For this review, take the finished solid that the model builds, in its own axes (mm). Coordinates: 2 decimals unless noted, no trailing zeros.
1) Insertion check: P1, Ø3, axis at y = -3.5, z = 3.5, coming from the -X side. The pin has a flat end and moves straight along its axis. Give the tip position at first contact, or say it passes through.
2) To check wall thickness, follow line 1 along X through (y, z) = (17, 6.75); line 2 along Y through (x, z) = (-6, 0.5); line 3 along Y through (x, z) = (45, 2.5). State the ranges of each line that lie inside material, in increasing order.
3) Mouldability with a two-part tool opening along X and no side actions: class faces 1 (the face through (-9, 15, 8)), 2 (the face through (-8.796, -0.004, 3.944)) as pulls with the +X half, pulls with the -X half, needs draft (parallel to the pull), parting line crosses it, or undercut.
from build123d import *

# Parameters (mm, degrees)
BOSS_EXTRU_2_DEPTH                 = 8
ENL_V_MAT_EXTRU_1_DEPTH            = 9
CONG_1_R                           = 10
R_P_TITION_CIRCULAIRE1_COUNT       = 9
R_P_TITION_CIRCULAIRE1_ANGLE       = 3.68
CONG_1_OF_R_P_TITION_CIRCULAIRE1_R = 10
R_P_TITION_CIRCULAIRE2_COUNT       = 9
R_P_TITION_CIRCULAIRE2_ANGLE       = 3.68
CONG_1_OF_R_P_TITION_CIRCULAIRE2_R = 10


with BuildPart() as part:
    # Esquisse1 → Boss.-Extru.2 (new body)
    with BuildSketch(Plane.XY):
        with BuildLine():
            Line((627.808263697, -21.923547662), (631.296087384, 27.954654851))
            ThreePointArc((631.296087384, 27.954654851), (0, 50), (-631.296087384, 27.954654851))
            Line((-631.296087384, 27.954654851), (-627.808263697, -21.923547662))
            ThreePointArc((-627.808263697, -21.923547662), (0, 0), (627.808263697, -21.923547662))
        make_face()
    extrude(amount=BOSS_EXTRU_2_DEPTH)

    # Esquisse2 → Enlèv. mat.-Extru.1 (cut, through all)
    with BuildSketch(Plane.XY.offset(8)):
        Polygon((0, 25), (30, 49.950276106), (0, 74.995327729), (-30, 49.950276106), align=None)
    enl_v_mat_extru_1 = extrude(amount=-ENL_V_MAT_EXTRU_1_DEPTH, mode=Mode.SUBTRACT)

    # Congé1
    cong_1_edges = [part.edges().sort_by_distance(p)[0] for p in [
        (0, 25, 4),
        (-30, 49.950276106, 4),
        (30, 49.950276106, 4),
    ]]
    fillet(cong_1_edges, radius=CONG_1_R)

    # Répétition circulaire1: Enlèv. mat.-Extru.1 ×9 about axis
    r_p_tition_circulaire1_axis = Axis((0, -9000, 0), (0, 0, 1))
    for i in range(1, R_P_TITION_CIRCULAIRE1_COUNT):
        add(enl_v_mat_extru_1.rotate(r_p_tition_circulaire1_axis, i * R_P_TITION_CIRCULAIRE1_ANGLE / (R_P_TITION_CIRCULAIRE1_COUNT - 1)), mode=Mode.SUBTRACT)

    # Congé1 of Répétition circulaire1
    cong_1_of_r_p_tition_circulaire1_edges = [part.edges().sort_by_distance(p)[0] for p in [
        (-72.456565501, 24.709139142, 4),
        (-102.655910154, 49.417758293, 4),
        (-42.657843855, 49.899463992, 4),
        (-144.908460692, 23.836575317, 4),
        (-175.305203447, 48.301944876, 4),
        (-115.312938126, 49.265325224, 4),
        (-217.351015561, 22.382364766, 4),
        (-247.943197144, 46.602907776, 4),
        (-187.960599706, 48.047900678, 4),
        (-289.779560701, 20.346601223, 4),
        (-320.565209242, 44.320756509, 4),
        (-260.596145965, 46.247268824, 4),
        (-362.189427606, 17.729415908, 4),
        (-393.166558764, 41.455638174, 4),
        (-333.214895057, 43.863545726, 4),
        (-434.575948977, 14.530977515, 4),
        (-465.742566067, 38.007737447, 4),
        (-405.812166217, 40.89688503, 4),
        (-506.934459016, 10.751492204, 4),
        (-538.288553142, 33.977276569, 4),
        (-478.383280064, 37.347477958, 4),
        (-579.260293733, 6.39120359, 4),
        (-610.799843913, 29.364515329, 4),
        (-550.923558903, 33.215553293, 4),
    ]]
    fillet(cong_1_of_r_p_tition_circulaire1_edges, radius=CONG_1_OF_R_P_TITION_CIRCULAIRE1_R)

    # Répétition circulaire2: Enlèv. mat.-Extru.1 ×9 about axis
    r_p_tition_circulaire2_axis = Axis((0, -9000, 0), (0, 0, -1))
    for i in range(1, R_P_TITION_CIRCULAIRE2_COUNT):
        add(enl_v_mat_extru_1.rotate(r_p_tition_circulaire2_axis, i * R_P_TITION_CIRCULAIRE2_ANGLE / (R_P_TITION_CIRCULAIRE2_COUNT - 1)), mode=Mode.SUBTRACT)

    # Congé1 of Répétition circulaire2
    cong_1_of_r_p_tition_circulaire2_edges = [part.edges().sort_by_distance(p)[0] for p in [
        (72.456565501, 24.709139142, 4),
        (42.657843855, 49.899463992, 4),
        (102.655910154, 49.417758293, 4),
        (144.908460692, 23.836575317, 4),
        (115.312938126, 49.265325224, 4),
        (175.305203447, 48.301944876, 4),
        (217.351015561, 22.382364766, 4),
        (187.960599706, 48.047900678, 4),
        (247.943197144, 46.602907776, 4),
        (289.779560701, 20.346601223, 4),
        (260.596145965, 46.247268824, 4),
        (320.565209242, 44.320756509, 4),
        (362.189427606, 17.729415908, 4),
        (333.214895057, 43.863545726, 4),
        (393.166558764, 41.455638174, 4),
        (434.575948977, 14.530977515, 4),
        (405.812166217, 40.89688503, 4),
        (465.742566067, 38.007737447, 4),
        (506.934459016, 10.751492204, 4),
        (478.383280064, 37.347477958, 4),
        (538.288553142, 33.977276569, 4),
        (579.260293733, 6.39120359, 4),
        (550.923558903, 33.215553293, 4),
        (610.799843913, 29.364515329, 4),
    ]]
    fillet(cong_1_of_r_p_tition_circulaire2_edges, radius=CONG_1_OF_R_P_TITION_CIRCULAIRE2_R)


solid = part.part
Result:
1. P1: stops at x = -629.2
2. line 1: x = -630.53 to -593.82, -568.05 to -515.37, -500.23 to 500.23, 515.37 to 568.05, 593.82 to 630.53
2. line 2: y = 0 to 30.01
2. line 3: y = -0.11 to 47.9
3. face 1: needs draft
3. face 2: undercut
